Design review of the part built by this model. Coordinates are the model's own, in mm. A direction names the side the tool comes from. Round coordinates to 2 decimals unless told otherwise and drop trailing zeros. Loops run counter-clockwise (first coordinate to the right, second up) from the corner with the lowest first, then second, coordinate; pieces in that order, holes last. Notation, with made-up numbers: M 8,38 L 28,38 A14 cw 28,59 Z; hole C -12,-24.75 d10. An arc over 180 degrees is marked long. One line per item, written item: value. Start each with the question number.
Item 1: For faces 4 (the flat face through (34, -2, -55.562)), 5 (the flat face through (-12.784, -1.503, -31.778)), list the 3-axis set-ups (+Z, -Z, +X, -X, +Y, -Y) from which the entire face can be reached by the end or side of a thin tool; tool diameter is ignored.
Item 2: Clearance check with flat-ended pins moving along their axes: pin 1 (1 mm diameter, centred on y = -0.5, z = -40, fed in from -X); pin 2 (1.5 mm diameter, centred on y = -2, z = -32, fed in from +X) (3 decimals); pin 3 (1.5 mm diameter, centred on x = 39, y = -2, fed in from +Z). State where each tip first meets the part, or that it passes through.
Item 3: For line 1 along Z through (x, y) = (-1, -2); line 2 along X through (y, z) = (-1.15, 53.5); line 3 along X through (y, z) = (-1.35, -41) (3 decimals), list the stretches that pass through material, from the lowest coordinate up.
Item 4: Mouldability with a two-part tool opening along Z and no side actions: class faces 1 (the cylindrical face through (-1.794, -1.503, 39.654)), 2 (the cylindrical face through (0.204, -1.503, 60.323)), 3 (the flat face through (3, 0, -20)) as released by +Z, released by -Z, zero draft, split by the parting line, or undercut.
Item 5: We need section B-B (z = -4). Write out the cut boundary in (x, y) (3 decimals).
Item 6: We need section C-C (x = 46). Write out the cut boundary in (y, z).
from build123d import *

# Parameters (mm, degrees)
F0_R     = 1.5875
F1_DEPTH = 3.048


with BuildPart() as f1:
    # F0 (on Front) → F1 (new body)
    with BuildSketch(Plane.XZ):
        with BuildLine():
            Line((0, 38.0796237513), (0, 41.275))
            ThreePointArc((0, 41.275), (-7.14375, 44.4998046905), (-9.4502929642, 51.990625))
            Line((-9.4502929642, 51.990625), (-15.7504883039, 1.9843747602))
            ThreePointArc((-15.7504883039, 1.9843747602), (-10.5003256064, 11.9062499201), (0, 15.875))
            Line((0, 15.875), (0, 38.0796237513))
        make_face()
        with Locations((-1.5875, 38.0796237513)):
            Circle(F0_R, mode=Mode.SUBTRACT)
        with BuildLine():
            ThreePointArc((9.525, 50.8), (6.7351920908, 44.0648079092), (0, 41.275))
            Line((0, 41.275), (0, 38.0796237513))
            Line((0, 38.0796237513), (0, 15.875))
            ThreePointArc((0, 15.875), (9.76389722, 12.5172655192), (15.3974543628, 3.8644565138))
            Line((15.3974543628, 3.8644565138), (9.4530967593, 51.9681552373))
            ThreePointArc((9.4530967593, 51.9681552373), (9.5070071956, 51.3851830343), (9.525, 50.8))
        make_face()
        with BuildLine():
            ThreePointArc((15.3974543628, 3.8644565138), (9.76389722, 12.5172655192), (0, 15.875))
            Line((0, 15.875), (0, -15.875))
            ThreePointArc((0, -15.875), (11.2253201513, -11.2253201513), (15.875, 0))
            Line((15.875, 0), (15.3974543628, 3.8644565138))
        make_face()
        with BuildLine():
            Line((0, -15.875), (0, 15.875))
            ThreePointArc((0, 15.875), (-10.5003256064, 11.9062499201), (-15.7504883039, 1.9843747602))
            ThreePointArc((-15.7504883039, 1.9843747602), (-11.9062499201, -10.5003256064), (0, -15.875))
        make_face()
        with BuildLine():
            ThreePointArc((15.875, 0), (11.2253201513, -11.2253201513), (0, -15.875))
            Line((0, -15.875), (0, -53.975))
            ThreePointArc((0, -53.975), (6.7351920908, -56.7648079092), (9.525, -63.5))
            Line((9.525, -63.5), (36.5125, -63.5))
            ThreePointArc((36.5125, -63.5), (38.8373399243, -57.8873399243), (44.45, -55.5625))
            Line((44.45, -55.5625), (23.8252, -55.5625))
            ThreePointArc((23.8252, -55.5625), (18.2035596682, -53.2339403318), (15.875, -47.6123))
            Line((15.875, -47.6123), (15.875, 0))
        make_face()
        with BuildLine():
            ThreePointArc((0, -15.875), (-11.9062499201, -10.5003256064), (-15.7504883039, 1.9843747602))
            Line((-15.7504883039, 1.9843747602), (-16.0004960241, 0))
            Line((-16.0004960241, 0), (-9.4765871109, -64.4591255022))
            ThreePointArc((-9.4765871109, -64.4591255022), (-7.0661621623, -57.1129054105), (0, -53.975))
            Line((0, -53.975), (0, -15.875))
        make_face()
        with BuildLine():
            ThreePointArc((9.525, -63.5), (6.7351920908, -56.7648079092), (0, -53.975))
            Line((0, -53.975), (0, -63.5))
            Line((0, -63.5), (9.525, -63.5))
        make_face()
        with BuildLine():
            Line((0, -63.5), (0, -53.975))
            ThreePointArc((0, -53.975), (-7.0661621623, -57.1129054105), (-9.4765871109, -64.4591255022))
            ThreePointArc((-9.4765871109, -64.4591255022), (-6.2598742362, -70.6791085482), (0.3401785714, -73.0189234444))
            ThreePointArc((0.3401785714, -73.0189234444), (6.8544082857, -70.1138273378), (9.525, -63.5))
            Line((9.525, -63.5), (0, -63.5))
        make_face()
        with BuildLine():
            Line((36.5125, -63.5), (9.525, -63.5))
            ThreePointArc((9.525, -63.5), (6.8544082857, -70.1138273378), (0.3401785714, -73.0189234444))
            Line((0.3401785714, -73.0189234444), (44.7334821429, -71.4324362036))
            ThreePointArc((44.7334821429, -71.4324362036), (38.9384772185, -69.2120069047), (36.5125, -63.5))
        make_face()
        with BuildLine():
            ThreePointArc((-9.4502929642, 51.990625), (-7.14375, 44.4998046905), (0, 41.275))
            ThreePointArc((0, 41.275), (6.7351920908, 44.0648079092), (9.525, 50.8))
            ThreePointArc((9.525, 50.8), (9.5070071956, 51.3851830343), (9.4530967593, 51.9681552373))
            ThreePointArc((9.4530967593, 51.9681552373), (0.0113220085, 60.324993271), (-9.4502929642, 51.990625))
        make_face()
        with BuildLine():
            ThreePointArc((44.45, -55.5625), (38.8373399243, -57.8873399243), (36.5125, -63.5))
            ThreePointArc((36.5125, -63.5), (38.9384772185, -69.2120069047), (44.7334821429, -71.4324362036))
            ThreePointArc((44.7334821429, -71.4324362036), (50.1620069047, -69.0115227815), (52.3875, -63.5))
            ThreePointArc((52.3875, -63.5), (50.0626600757, -57.8873399243), (44.45, -55.5625))
        make_face()
    extrude(amount=F1_DEPTH)


solid = f1.part
A:
1. face 4: +Z, +X, +Y, -Y
1. face 5: -Z, -X, +Y, -Y
2. pin 1: x = -12
2. pin 2: x = 15.875
2. pin 3: z = -55.56
3. line 1: -72.97 to 36.6, 39.55 to 60.27
3. line 2: -9.13 to 9.13
3. line 3: -11.851 to 15.875
4. face 1: undercut
4. face 2: released by +Z
4. face 3: zero draft
5. outline: M -15.596,-3.048 L 15.875,-3.048 L 15.875,0 L -15.596,0 Z
6. outline: M -3.05,-71.28 L 0,-71.28 L 0,-55.72 L -3.05,-55.72 Z
